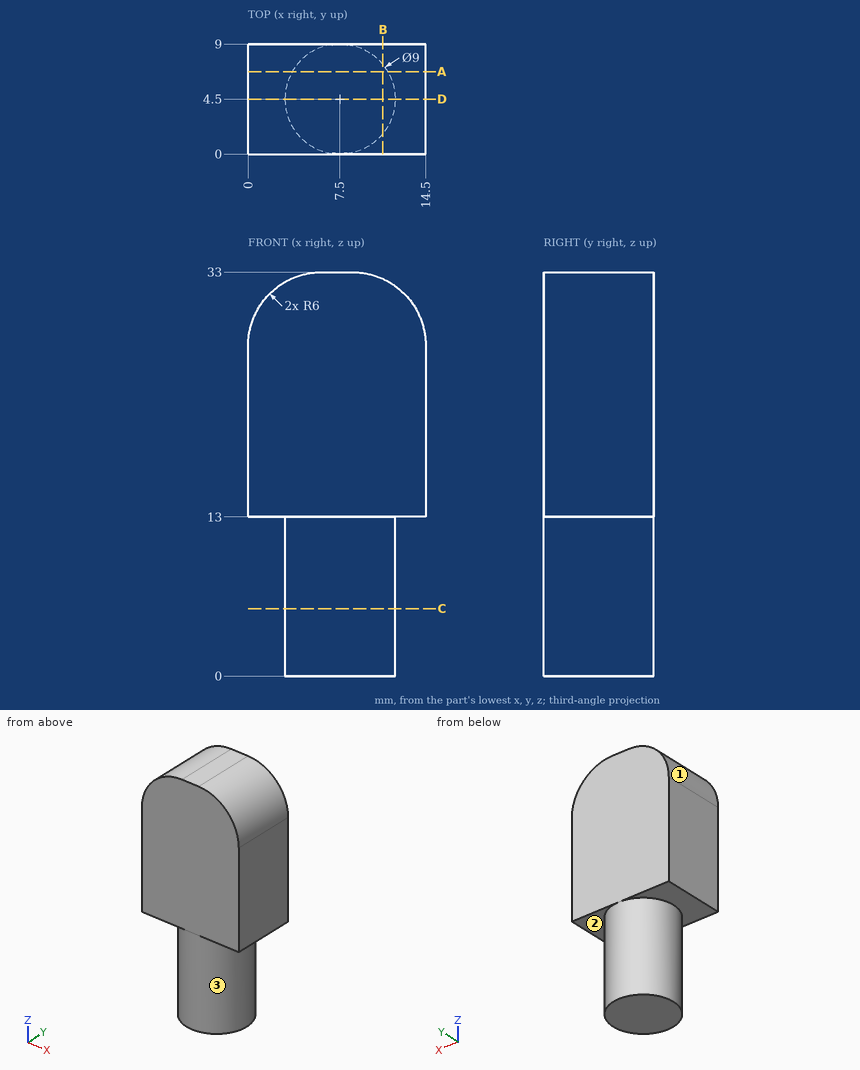
Geometry check sheet. Reference: drawing and pictorial views, mm from the part's lowest x, y, z. A direction names the side the tool comes from. Round coordinates to 2 decimals unless told otherwise and drop trailing zeros. Loops run counter-clockwise (first coordinate to the right, second up) from the corner with the lowest first, then second, coordinate; pieces in that order, holes last. Notation, with made-up numbers: (57.25, -17.5) -> (114.25, -17.5) arc R28 ccw to (114.25, 1.5) -> close; hole circle Ø4 at (-37, 11.25). An arc over 180 degrees is marked (long way). Answer as a JSON object with one key per item and string values. Group by question number.
Item 1: Thickness scan on line 1 along Y through (x, z) = (6.25, 3); line 2 along X through (y, z) = (8.5, 3); line 3 along Z through (x, y) = (2.25, 4.25). Record the ranges inside material, lowest first.
Item 2: Set-up check for the marked faces 1, 2 and 3: record each of +Z, -Z, +X, -X, +Y, -Y from which the full face is reachable in a straight line by a thin tool's end or side.
Item 3: Cross-section at A-A, the plane y = 6.75. Record the cut outline in (x, z).
Item 4: Cross-section at D-D, the plane y = 4.5. Record the cut outline in (x, z), plus the area to 3 significant figures.
Item 5: Cross-section at B-B, the plane x = 11. Record the cut outline in (y, z), plus the area to 3 significant figures.
Item 6: Cross-section at C-C, the plane z = 5.5. Record the cut outline in (x, y).
Item 7: Depth check by flat-ended pin: pin 1 Ø4 at (y, z) = (7, 5) entering from +X; pin 2 Ø4 at (x, y) = (3, 3.5) entering from +Z. Enter the tip coordinate at first touch or a pass-through.
Determined:
{
 "1": {"line 1": "y = 0.18 to 8.82", "line 2": "x = 5.44 to 9.56", "line 3": "z = 13 to 31.68"},
 "2": {"face 1": "+Z, -X, +Y, -Y", "face 2": "-Z, +X", "face 3": "-Z"},
 "3": {"outline": "(0, 13) -> (3.6, 13) -> (3.6, 0) -> (11.4, 0) -> (11.4, 13) -> (14.5, 13) -> (14.5, 27) arc R6 ccw to (8.5, 33) -> (6, 33) arc R6 ccw to (0, 27) -> close"},
 "4": {"outline": "(0, 13) -> (3, 13) -> (3, 0) -> (12, 0) -> (12, 13) -> (14.5, 13) -> (14.5, 27) arc R6 ccw to (8.5, 33) -> (6, 33) arc R6 ccw to (0, 27) -> close", "area": "392 mm²"},
 "5": {"outline": "(0, 13) -> (1.67, 13) -> (1.67, 0) -> (7.33, 0) -> (7.33, 13) -> (9, 13) -> (9, 32.45) -> (0, 32.45) -> close", "area": "249 mm²"},
 "6": {"outline": "circle Ø9 at (7.5, 4.5)"},
 "7": {"pin 1": "stops at x = 11.97", "pin 2": "stops at z = 32.92"}
}
